```python
from build123d import *

# Parameters (mm, degrees)
F0_W     = 381
F0_H     = 762
F0_W_2   = 254
F0_H_2   = 635
F1_DEPTH = 374.65
F2_DEPTH = 6.35


# Not quite as in the source:
# - a feature names something its author has since deleted; it is built from what else it names


with BuildPart() as f1:
    # F0 (on Front) → F1 (new body)
    with BuildSketch(Plane.XZ):
        with Locations((73.4267770052, 381)):
            Rectangle(F0_W, F0_H)
        with Locations((73.4267770052, 381)):
            Rectangle(F0_W_2, F0_H_2, mode=Mode.SUBTRACT)
        with Locations((73.4267770052, 381)):
            Rectangle(F0_W_2, F0_H_2)
    extrude(amount=-F1_DEPTH)

    # F0 (on Front) → F2 (cut)
    with BuildSketch(Plane.XZ):
        with Locations((73.4267770052, 381)):
            Rectangle(F0_W_2, F0_H_2)
    extrude(amount=-F2_DEPTH, mode=Mode.SUBTRACT)


solid = f1.part
```
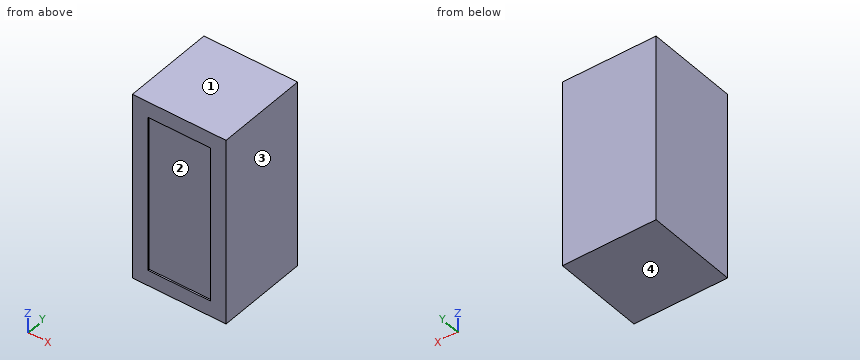
Geometry check sheet. Reference: the model listing, model coordinates, mm. Face numbers are marked on the shaded views. Give positions to 0.01 mm unless a question says otherwise; leave off trailing zeros. Write item = value, one per line. Start each with the question number.
1. Draft check along Z on the marked faces 1, 2, 3 and 4. Enter one of: +Z half, -Z half, draft (parallel to the pull), parting line (faces both ways), or undercut.
2. Thickness scan on probe 1 along Y at (x, z) = (152, 85.5). Record the ranges inside material, lowest first.
3. Go/stop test with flat-tipped pins: P1, Ø6, axis at x = 30.5, y = 254.5, coming from the -Z side; P2, Ø6, axis at x = 133.5, z = 128.5, coming from the -Y side. Record where each tip stops, or that it passes through.
Values follow:
q1.face_1 = +Z half
q1.face_2 = undercut
q1.face_3 = draft
q1.face_4 = -Z half
q2.probe_1 = 6.35 to 374.65
q3.P1 = 0
q3.P2 = 6.35
